Source: CAD feature listing. Evaluate the final solid. Frame: model axes, mm. A direction names the side the tool comes from. Round coordinates to 2 decimals unless told otherwise and drop trailing zeros. Write each loop counter-clockwise with the first axis right and the second up, starting at its lowest first coordinate (ties: lowest second). Pieces come first, ordered by that corner, then holes. Notation, with made-up numbers: M -20.75,-25 L -12.75,-25 A25 cw -12.75,13 Z; hole C -35,-36.75 d1. An arc over 180 degrees is marked long. Answer in a Markdown table with one row per item.
from build123d import *

# Parameters (mm, degrees)
BOSS_EXTRUDE1_DEPTH = 5
SKETCH2_R           = 1
CUT_EXTRUDE1_DEPTH  = 5
FILLET1_R           = 1


with BuildPart() as part:
    # Sketch1 → Boss-Extrude1 (new body)
    with BuildSketch(Plane(origin=(0, 0, 0), x_dir=(1, 0, 0), z_dir=(0, 1, 0))):
        Polygon((0, 0), (0, 6), (16.608456475, 6), (20, 6), (20, 4), (10, 4), (10, 0), align=None)
    extrude(amount=BOSS_EXTRUDE1_DEPTH)

    # Sketch2 → Cut-Extrude1 (cut)
    with BuildSketch(Plane.XY.offset(-4)):
        with Locations((12.523987241, 2.5)):
            Circle(SKETCH2_R)
        with Locations((18.223987241, 2.5)):
            Circle(SKETCH2_R)
    extrude(amount=-CUT_EXTRUDE1_DEPTH, mode=Mode.SUBTRACT)

    # Fillet1
    fillet1_edges = [part.edges().sort_by_distance(p)[0] for p in [
        (5, 0, 0),
        (5, 5, 0),
        (0, 5, -3),
        (10, 5, -6),
        (20, 5, -5),
        (15, 5, -4),
        (10, 5, -2),
        (0, 2.5, 0),
        (10, 2.5, 0),
        (10, 0, -2),
        (10, 0, -6),
        (15, 0, -4),
    ]]
    fillet(fillet1_edges, radius=FILLET1_R - 0.0001)  # a hair under: the kernel refuses the full size


solid = part.part
Q1. Section B-B (z = -2.7). Return loops of the section in (x, y).
Solutions:
| item | result |
|---|---|
| outline | M 0,0 L 9,0 A1 ccw 10,1 L 10,4 A1 ccw 9,5 L 1,5 A1 ccw 0,4 Z |
Q2. Section C-C (y = 1.3). Return loops of the section in (x, z), and give its area (3 significant figures).
Solutions:
| item | result |
|---|---|
| outline | M 0,-6 L 20,-6 L 20,-4 L 10,-4 L 10,-1 A1 ccw 9,0 L 1,0 A1 ccw 0,-1 Z |
| area | 79.6 mm2 |
Q3. Access query for faces 4 (the cylindrical face through (9.699, 4.715, -2.527)), 5 (the cylindrical face through (0.285, 2.028, -0.301)), 6 (the flat face through (3, 0, -3)), 7 (the cylindrical face through (14.423, 0.285, -4.301)), 8 (the flat face through (10, 2, -3)). Directions: +Z, -Z, +X, -X, +Y, -Y. A direction counts if a zero-diameter tool reaches every point of the face in a straight line with its end or side. Return the directions, or none.
Solutions:
| item | result |
|---|---|
| face 4 | +Z, +X, +Y |
| face 5 | +Z, -X, +Y, -Y |
| face 6 | +Z, -Z, +X, -X, -Y |
| face 7 | +Z, +X, -Y |
| face 8 | +Z, +X, +Y, -Y |
Q4. Pull-direction query (X, two-part tool) for faces 1 (the cylindrical face through (9.86, 4.699, -5.715)), 2 (the cylindrical face through (11.525, 2.544, -4.986)), 3 (the flat face through (20, 2, -5)); classes: pulls with the +X half, pulls with the -X half, needs draft (parallel to the pull), parting line crosses it, or undercut.
Solutions:
| item | result |
|---|---|
| face 1 | needs draft |
| face 2 | undercut |
| face 3 | pulls with the +X half |
Q5. Section D-D (x = 8.25). Return loops of the section in (y, z).
Solutions:
| item | result |
|---|---|
| outline | M 0,-5 A1 ccw 1,-6 L 4,-6 A1 ccw 5,-5 L 5,-1 A1 ccw 4,0 L 1,0 A1 ccw 0,-1 Z |
Q6. Section A-A (y = 2.5). Return loops of the section in (x, z).
Solutions:
| item | result |
|---|---|
| outline | M 0,-6 L 11.52,-6 L 11.52,-4 L 10,-4 L 10,-1 A1 ccw 9,0 L 1,0 A1 ccw 0,-1 Z; M 13.52,-6 L 17.22,-6 L 17.22,-4 L 13.52,-4 Z; M 19.22,-6 L 20,-6 L 20,-4 L 19.22,-4 Z |
Q7. Material intervals for probe 1 along Y at (x, z) = (12.5, -4.95); probe 2 along Z at (x, y) = (14.25, 1.25); probe 3 along Z at (x, y) = (3, 0.75), sorted ascending.
Solutions:
| item | result |
|---|---|
| probe 1 | y = 0 to 1.5, 3.5 to 5 |
| probe 2 | z = -6 to -4 |
| probe 3 | z = -5.97 to -0.03 |
Q8. Contact query for flat-ended pins moving along their axis: pin 1 Ø1.5 at (y, z) = (2.5, -3) entering from +X; pin 2 Ø0.9 at (x, y) = (14.5, 2) entering from +Z. Output: stop coordinate, or through.
Solutions:
| item | result |
|---|---|
| pin 1 | stops at x = 10 |
| pin 2 | stops at z = -4 |
